Design review of the part built by this model. Coordinates are the model's own, in mm. Face numbers are marked on the shaded views. A direction names the side the tool comes from. Coordinates: 2 decimals unless noted, no trailing zeros. Write each loop counter-clockwise with the first axis right and the second up, starting at its lowest first coordinate (ties: lowest second). Pieces come first, ordered by that corner, then holes. Notation, with made-up numbers: (14, -29) - (66, -29) arc R34 ccw to (66, 1) - close; hole circle Ø7 at (42, 20). An arc over 180 degrees is marked (long way). Use a Markdown table: item, result.
Autodesk Inventor part; units mm, degrees
ref_plane "YZ Plane" through (0, 0, 0) normal (1, 0, 0) x (0, 1, 0)
ref_plane "XZ Plane" through (0, 0, 0) normal (0, 1, 0) x (-1, 0, 0)
ref_plane "XY Plane" through (0, 0, 0) normal (0, 0, 1) x (1, 0, 0)
sketch "Sketch1" plane through (0, 0, 0) normal (0, 0, 1) x (1, 0, 0)
  line L0 (0, 0) -> (11.1125, 0)
  line L1 (11.1125, 0) -> (11.1125, 6.35)
  line L2 (3.175, 26.9748) -> (0, 26.9748)
  line L3 (0, 26.9748) -> (0, 0)
  line L4 (3.175, 26.9748) -> (3.175, 12.7)
  line L5 (3.175, 12.7) -> (7.9502, 12.7)
  line L6 (7.9502, 12.7) -> (7.9502, 6.35)
  line L7 (7.9502, 6.35) -> (11.1125, 6.35)
  dimension "d2" = 3.175
  dimension "d3" = 7.9502
revolve "Revolution1" add sketch "Sketch1" angle 360 about axis through (0, 26.9748, 0) along (0, -1, 0)
fillet "Fillet1" radius 7.9248 1 edges at (-7.9502, 6.35, 0)
chamfer "Chamfer1" distance 1.524 angle 45 1 edges at (-11.1125, 0, 0)
properties part number "Rack Pad" material "Stainless Steel"
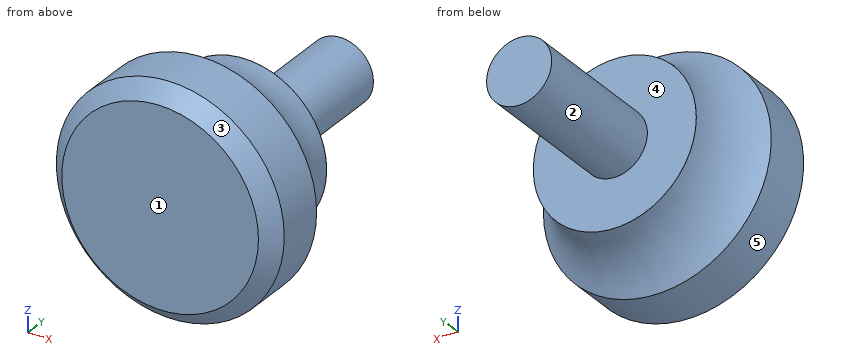
(1) For L1, parallel to Y at x = 1.5, z = 4.5; L2, parallel to Z at x = -0.5, y = 11; L3, parallel to X at y = 8.25, z = 5.75, list the stretches that pass through material, from the lowest coordinate up. Write a range as from..to.
Determined:
| item | result |
|---|---|
| L1 | 0..12.7 |
| L2 | -8.12..8.12 |
| L3 | -7.32..7.32 |
(2) Machinability: for the marked faces 1 and 2, which of the approach directions +Z, -Z, +X, -X, +Y, -Y give a long, thin tool a straight path to every point of the face, cutting with its end or side? Answer none if there is none.
Determined:
| item | result |
|---|---|
| face 1 | +Z, -Z, +X, -X, -Y |
| face 2 | +Y |
(3) Take a section at D-D on y = 5.25. Write out the cut boundary in (x, z) (1 decimal).
Determined:
| item | result |
|---|---|
| outline | circle Ø22.2 at (0, 0) |
(4) For pin 1 (1 mm diameter, centred on x = -3, y = 20.5, fed in from +Z); pin 2 (2 mm diameter, centred on y = 16, z = 0, fed in from -X) (3 decimals); pin 3 (6 mm diameter, centred on x = -0.5, y = 23, fed in from -Z) (3 decimals), all flat-tipped, find the tip position at first contact; note any pin that passes through.
Determined:
| item | result |
|---|---|
| pin 1 | z = 1.96 |
| pin 2 | x = -3.175 |
| pin 3 | z = -3.175 |
(5) Take a section at C-C on y = 25. Write out the cut boundary in (x, z) (3 decimals).
Determined:
| item | result |
|---|---|
| outline | circle Ø6.35 at (0, 0) |
(6) Draft analysis for pull direction Y (two halves, no side actions). For the marked faces 3, 4 and 5, state which applies: +Y half, -Y half, draft (parallel to the pull), parting line (faces both ways), or undercut.
Determined:
| item | result |
|---|---|
| face 3 | -Y half |
| face 4 | +Y half |
| face 5 | draft |
